Verification items for the finished model (mm, model axes). A direction names the side the tool comes from. Round coordinates to 2 decimals unless told otherwise and drop trailing zeros. Order: outer loops, then holes, each group sorted by start corner. A loop starts at its lowest first (then second) coordinate and runs counter-clockwise, first axis right, second up. Notation, with made-up numbers: (16.25, 63.5) -> (52.25, 63.5) arc R26 ccw to (52.25, 88.5) -> close; hole circle Ø4 at (9, 2.5). An arc over 180 degrees is marked (long way). Return JSON: item names as keys, results as strings. Group by question number.
1) Section check D-D on y = 26.25. Enter the section's corners in (x, z).
2) Scan lines: L1, parallel to X at y = 28.55, z = 0; L2, parallel to X at y = 20.5, z = -0.25; L3, parallel to Y at x = -3, z = -3. Record each from-to range of solid material in increasing order.
3) Depth check by flat-ended pin: pin 1 (0.9 mm diameter, centred on x = 16.5, z = -2, fed in from -Y); pin 2 (8 mm diameter, centred on x = -9.5, z = -1, fed in from +Y); pin 3 (2 mm diameter, centred on y = 21.5, z = 2.5, fed in from +X). Enter the tip coordinate at first touch or a pass-through.
4) Section check A-A on x = 16.5. Enter the section's corners in (y, z).
5) Tool access check on faces 1 (the cylindrical face through (12.483, 28.986, -0.26)), 2 (the flat face through (16.658, 26.014, -2.564)), 3 (the flat face through (17.4, 26, 0.8)). Record the directions out of +Z, -Z, +X, -X, +Y, -Y that give a thin tool (end or side, any length) a straight path to the whole face; none if there is none.
6) Draft check along X on faces 4 (the cylindrical face through (11.132, 29.014, 0.403)), 5 (the cylindrical face through (15.3, 26, -3.3)), 6 (the flat face through (0, 13, -7.5)), 7 (the flat face through (11, 28, 0)). Enter one of: pulls with the +X half, pulls with the -X half, needs draft (parallel to the pull), parting line crosses it, or undercut.
```python
from build123d import *

# Parameters (mm, degrees)
SKETCH1_W           = 30
SKETCH1_H           = 15
BOSS_EXTRUDE1_DEPTH = 27
SKETCH8_W           = 27
SKETCH8_H           = 12
BOSS_EXTRUDE5_DEPTH = 1
FILLET4_R           = 1
SKETCH9_R           = 2
BOSS_EXTRUDE6_DEPTH = 2
SKETCH10_R          = 0.75
CUT_EXTRUDE2_DEPTH  = 2
BOSS_EXTRUDE7_DEPTH = 2
FILLET5_R           = 1


# Some blends are built 0.0001 mm under size
with BuildPart() as part:
    # Sketch1 → Boss-Extrude1 (new body)
    with BuildSketch(Plane(origin=(0, 0, 0), x_dir=(1, 0, 0), z_dir=(0, 1, 0))):
        Rectangle(SKETCH1_W, SKETCH1_H)
    extrude(amount=BOSS_EXTRUDE1_DEPTH)

    # Sketch8 → Boss-Extrude5 (add)
    with BuildSketch(Plane(origin=(0, 27, 0), x_dir=(1, 0, 0), z_dir=(0, 1, 0))):
        Rectangle(SKETCH8_W, SKETCH8_H)
    extrude(amount=BOSS_EXTRUDE5_DEPTH)

    # Fillet4
    fillet4_edges = [part.edges().sort_by_distance(p)[0] for p in [
        (0, 27, 6),
        (13.5, 27, 0),
        (-13.5, 27, 0),
        (0, 27, -6),
    ]]
    fillet(fillet4_edges, radius=FILLET4_R - 0.0001)  # a hair under: the kernel refuses the full size

    # Sketch9 → Boss-Extrude6 (add)
    with BuildSketch(Plane(origin=(0, 28, 0), x_dir=(1, 0, 0), z_dir=(0, 1, 0))):
        with Locations(Location((10.5, 0, 0), (0, 0, 270))):
            Circle(SKETCH9_R)
    extrude(amount=BOSS_EXTRUDE6_DEPTH)

    # Sketch10 → Cut-Extrude2 (cut)
    with BuildSketch(Plane(origin=(0, 30, 0), x_dir=(1, 0, 0), z_dir=(0, 1, 0))):
        with Locations(Location((10.5, 0, 0), (0, 0, 270))):
            Circle(SKETCH10_R)
    extrude(amount=-CUT_EXTRUDE2_DEPTH, mode=Mode.SUBTRACT)

    # Sketch11 → Boss-Extrude7 (add)
    with BuildSketch(Plane(origin=(0, 27, 0), x_dir=(1, 0, 0), z_dir=(0, 1, 0))):
        with BuildLine():
            Line((15, 3.017710153), (15.890097225, 3.017710153))
            Line((15.890097225, 3.017710153), (17.939578486, 1.806653045))
            Line((17.939578486, 1.806653045), (17.939578486, 0.8))
            Line((17.939578486, 0.8), (16.914837856, 0.8))
            ThreePointArc((16.914837856, 0.8), (16.114837856, 0), (16.914837856, -0.8))
            Line((16.914837856, -0.8), (17.939578486, -0.8))
            Line((17.939578486, -0.8), (17.939578486, -1.806653045))
            Line((17.939578486, -1.806653045), (15.890097225, -3.017710153))
            Line((15.890097225, -3.017710153), (15, -3.017710153))
            Line((15, -3.017710153), (15, 3.017710153))
        make_face()
    extrude(amount=-BOSS_EXTRUDE7_DEPTH)

    # Fillet5
    # the kernel refuses this fillet: 1 mm, written as the material it adds along each edge
    with BuildSketch(Plane(origin=(15, 27, 3.017710153), x_dir=(0, 0, 1), z_dir=(0, -1, 0))) as fillet5_piece_1:
        with BuildLine():
            CenterArc((0.993942342, -1), FILLET5_R, 90, 83.690289012)
            Line((0, -0.890097225), (0, 0))
            Line((0, 0), (0.993942342, 0))
        make_face()
    extrude(amount=2)
    with BuildSketch(Plane(origin=(15, 27, -3.017710153), x_dir=(0, 0, -1), z_dir=(0, -1, 0))) as fillet5_piece_2:
        with BuildLine():
            CenterArc((0.993942342, 1), FILLET5_R, 186.309710988, 83.690289012)
            Line((0, 0.890097225), (0, 0))
            Line((0, 0), (0.993942342, 0))
        make_face()
    extrude(amount=2)
    # the kernel refuses this fillet: 1 mm, written as the material it takes off along each edge
    with BuildSketch(Plane(origin=(17.939578486, 28.426575532, -1.806653045), x_dir=(0, 0, 1), z_dir=(0, -1, 0)), Plane(origin=(17.939578486, 28.426575532, 1.806653045), x_dir=(-0.8609265282144232, 0, 0.5087293121264587), z_dir=(0, -1, 0))) as fillet5_2_piece_1:
        with BuildLine():
            CenterArc((FILLET5_R * 0.570630212653, FILLET5_R), FILLET5_R, 210.579226872, 59.420773128)
            Line((-FILLET5_R * 0.290296315561, FILLET5_R * 0.491270687874), (0, 0))
            Line((0, 0), (FILLET5_R * 0.570630212653, 0))
        make_face()
    extrude(amount=4.853151063, mode=Mode.SUBTRACT)


solid = part.part
```
Check result:
{
 "1": {"outline": "(-15, -7.5) -> (15, -7.5) -> (15, -4.01) arc R1 cw to (15.89, -3.02) -> (17.45, -2.1) arc R1 ccw to (17.94, -1.24) -> (17.94, -0.8) -> (16.91, -0.8) arc R0.8 cw to (16.91, 0.8) -> (17.94, 0.8) -> (17.94, 1.24) arc R1 ccw to (17.45, 2.1) -> (15.89, 3.02) arc R1 cw to (15, 4.01) -> (15, 7.5) -> (-15, 7.5) -> close"},
 "2": {"L1": "8.5 to 9.75, 11.25 to 12.5", "L2": "-15 to 15", "L3": "0 to 28"},
 "3": {"pin 1": "y = 25", "pin 2": "y = 28", "pin 3": "x = 15"},
 "4": {"outline": "(25, -2.66) -> (27, -2.66) -> (27, -0.68) -> (25, -0.68) -> close; (25, 0.68) -> (27, 0.68) -> (27, 2.66) -> (25, 2.66) -> close"},
 "5": {"face 1": "+Y", "face 2": "-Z, +X, +Y, -Y", "face 3": "+X, +Y, -Y"},
 "6": {"face 4": "undercut", "face 5": "pulls with the +X half", "face 6": "needs draft", "face 7": "undercut"}
}
